For this review, take the finished solid that the model builds, in its own axes (mm). A direction names the side the tool comes from. Give positions to 0.01 mm unless a question says otherwise; leave off trailing zeros. Write each loop counter-clockwise with the first axis right and the second up, starting at its lowest first coordinate (ties: lowest second). Pieces come first, ordered by that corner, then holes. Notation, with made-up numbers: M 39,34.5 L 57,34.5 A20 ccw 57,56.5 Z; hole C 65.25,41 d11. An arc over 180 degrees is marked long. Use one line per item in the form item = value. Start each with the question number.
Q1. Clearance check with flat-ended pins moving along their axes: pin 1 Ø1 at (x, z) = (0.5, 43.5) entering from -Y; pin 2 Ø1.1 at (x, z) = (0.5, 14) entering from -Y; pin 3 Ø5 at (y, z) = (1.5, 26.5) entering from +X. State where each tip first meets the part, or that it passes through.
Q2. For probe 1 along Z at (x, y) = (1.5, 2.5); probe 2 along Z at (x, y) = (3.5, -1.5); probe 3 along Y at (x, z) = (-1.5, 9), list the stretches that pass through material, from the lowest coordinate up. Write a range as [from, to].
Q3. Consider section C-C on z = 36. Write out the cut boundary in (x, y).
Q4. Tool access review of faces 1 (the flat face through (-2.79, -1.58, 12.62)), 2 (the flat face through (1, 4, 5)), 3 (the flat face through (2.37, -1.394, 44.33)), 4 (the flat face through (-2.37, 1.394, 44.33)), 5 (the flat face through (3.3, -1, 7)): name each direction out of +Z, -Z, +X, -X, +Y, -Y from which nothing blocks a thin tool from reaching the whole face with its end or side.
Q5. Consider section B-B on z = 8.5. Write out the cut boundary in (x, y), and give its area (3 significant figures).
Q6. Consider section A-A on z = 44.5. Write out the cut boundary in (x, y) (1 decimal).
```python
from build123d import *

# Parameters (mm, degrees)
SKETCH1_R           = 3.75
BOSS_EXTRUDE1_DEPTH = 5
SKETCH2_R           = 5
BOSS_EXTRUDE2_DEPTH = 2
BOSS_EXTRUDE3_DEPTH = 11.4
SKETCH4_R           = 3.204293994
BOSS_EXTRUDE4_DEPTH = 21
BOSS_EXTRUDE5_DEPTH = 10
SKETCH6_R           = 2.749630657
BOSS_EXTRUDE6_DEPTH = 5


with BuildPart() as part:
    # Sketch1 → Boss-Extrude1 (new body)
    with BuildSketch(Plane.XY):
        Circle(SKETCH1_R)
    extrude(amount=BOSS_EXTRUDE1_DEPTH)

    # Sketch2 → Boss-Extrude2 (add)
    with BuildSketch(Plane.XY.offset(5)):
        Circle(SKETCH2_R)
    extrude(amount=BOSS_EXTRUDE2_DEPTH)

    # Sketch3 → Boss-Extrude3 (add)
    with BuildSketch(Plane.XY.offset(7)):
        Polygon((3.7, 0), (1.85, 3.204293994), (-1.85, 3.204293994), (-3.7, 0), (-1.85, -3.204293994), (1.85, -3.204293994), align=None)
    extrude(amount=BOSS_EXTRUDE3_DEPTH)

    # Sketch4 → Boss-Extrude4 (add)
    with BuildSketch(Plane.XY.offset(18.4)):
        Circle(SKETCH4_R)
    extrude(amount=BOSS_EXTRUDE4_DEPTH)

    # Sketch5 → Boss-Extrude5 (add)
    with BuildSketch(Plane.XY.offset(39.4)):
        Polygon((3.175, 0), (1.5875, 2.749630657), (-1.5875, 2.749630657), (-3.175, 0), (-1.5875, -2.749630657), (1.5875, -2.749630657), align=None)
    extrude(amount=BOSS_EXTRUDE5_DEPTH)

    # Sketch6 → Boss-Extrude6 (add)
    with BuildSketch(Plane.XY.offset(49.4)):
        Circle(SKETCH6_R)
    extrude(amount=BOSS_EXTRUDE6_DEPTH)


solid = part.part
```
Working result:
q1.pin_1 = -2.75
q1.pin_2 = -3.2
q1.pin_3 = 3.2
q2.probe_1 = [0, 49.4]
q2.probe_2 = [5, 7]
q2.probe_3 = [-3.2, 3.2]
q3.outline = C 0,0 d6.41
q4.face_1 = +Z, -X, -Y
q4.face_2 = -Z
q4.face_3 = +Z, +X, -Y
q4.face_4 = +Z, -X, +Y
q4.face_5 = +Z
q5.outline = M -3.7,0 L -1.85,-3.2 L 1.85,-3.2 L 3.7,0 L 1.85,3.2 L -1.85,3.2 Z
q5.area = 35.6 mm²
q6.outline = M -3.2,0 L -1.6,-2.7 L 1.6,-2.7 L 3.2,0 L 1.6,2.7 L -1.6,2.7 Z
